from build123d import *

# Parameters (mm, degrees)
SKETCH_1_W          = 19
SKETCH_1_H          = 32
EXTRUDE_1_DEPTH     = 67
FILLET_1_R          = 1
SHELL_1_T           = 1.3
SKETCH_2_W          = 49
SKETCH_2_H          = 24
CUT_EXTRUDE_1_DEPTH = 74.32305231
CUT_EXTRUDE_2_REACH = 79.322
SKETCH_4_W          = 5.786103887
SKETCH_4_H          = 2
SKETCH_4_W_2        = 5.809063148
EXTRUDE_2_DEPTH     = 1.3


with BuildPart() as part:
    # 草图1 → 凸台-拉伸1 (new body)
    with BuildSketch(Plane(origin=(0, 0, 0), x_dir=(0, 0, -1), z_dir=(1, 0, 0))):
        Rectangle(SKETCH_1_W, SKETCH_1_H)
    extrude(amount=EXTRUDE_1_DEPTH)

    # 圆角1
    fillet_1_edges = [part.edges().sort_by_distance(p)[0] for p in [
        (67, -16, 0),
        (0, -16, 0),
        (0, 16, 0),
        (67, 16, 0),
    ]]
    fillet(fillet_1_edges, radius=FILLET_1_R)

    # 抽壳1
    shell_1_openings = [part.faces().sort_by_distance(p)[0] for p in [
        (33.5, 0, -9.5),
    ]]
    offset(amount=SHELL_1_T, openings=shell_1_openings, kind=Kind.INTERSECTION)

    # 草图2 → 切除-拉伸1 (cut, through all)
    with BuildSketch(Plane.XY.offset(10.8)):
        with Locations((32, 0)):
            Rectangle(SKETCH_2_W, SKETCH_2_H)
    extrude(amount=-CUT_EXTRUDE_1_DEPTH, mode=Mode.SUBTRACT)

    # 草图3 → 切除-拉伸2 (cut, up to next)
    with BuildSketch(Plane.XZ.offset(17.3), mode=Mode.PRIVATE) as cut_extrude_2_sk1:
        with BuildLine():
            Line((11.05, 2.9), (17.35, 2.9))
            ThreePointArc((17.35, 2.9), (19.1, 1.15), (17.35, -0.6))
            Line((17.35, -0.6), (11.05, -0.6))
            ThreePointArc((11.05, -0.6), (9.3, 1.15), (11.05, 2.9))
        make_face()
    cut_extrude_2_tool1 = extrude(cut_extrude_2_sk1.sketch, amount=-CUT_EXTRUDE_2_REACH, mode=Mode.PRIVATE) & part.part
    add(cut_extrude_2_tool1.solids().sort_by_distance((14.2, -17.3, 1.15))[0], mode=Mode.SUBTRACT)

    # 草图4 → 凸台-拉伸2 (add)
    with BuildSketch(Plane.XZ.offset(-16)):
        with Locations((10.323725872, 2)):
            Rectangle(SKETCH_4_W, SKETCH_4_H)
        with Locations((58.142746149, 2)):
            Rectangle(SKETCH_4_W_2, SKETCH_4_H)
    extrude(amount=EXTRUDE_2_DEPTH)


solid = part.part
Can you work these out from the model? Positions are in its coordinate system, mm. A direction names the side the tool comes from. Round coordinates to 2 decimals unless told otherwise and drop trailing zeros. Write each loop counter-clockwise with the first axis right and the second up, starting at its lowest first coordinate (ties: lowest second). Pieces come first, ordered by that corner, then holes. Notation, with made-up numbers: (69.5, 48) -> (110.5, 48) arc R17 ccw to (110.5, 53) -> close; hole circle Ø6 at (-9, 40.25). An arc over 180 degrees is marked (long way). Use one line per item in the form item = value. Start each with the question number.
Q1. Imagine slicing it at C-C (x = 62). Please give me the cut outline in (y, z), then the cut area to 3 significant figures.
Q2. We'd pull the mould along Y, two halves only. Please class faces 6 (the face through (10, 14.7, 2)), 7 (the face through (68.3, 0, 1)), 8 (the face through (33, -17.3, 1)): +Y half, -Y half, draft (parallel to the pull), parting line (faces both ways), or undercut.
Q3. Imagine slicing it at B-B (y = -9). Please give me the cut outline in (x, z).
Q4. If I drill on probe 1 along Y at (x, z) = (52, 10.25); probe 2 along Y at (x, z) = (14.5, -2.5); probe 3 along X at (y, z) = (7, -2.75), over which ranges is the centre line in solid material (lowest first)? Write a range as [from, to].
Q5. Imagine slicing it at D-D (z = 6.5). Please give me the cut outline in (x, y).
Q6. Imagine slicing it at A-A (x = 46). Please give me the cut outline in (y, z), then the cut area to 3 significant figures.
Q7. Which directions (+Z, -Z, +X, -X, +Y, -Y) give clear straight access to the entire face, cutting with the end or side of a thin tool? Please do faces 1 (the face through (32, -12, 10)), 2 (the face through (23, 17, -9.5)), 3 (the face through (33, 17.3, 1)), 4 (the face through (33, -16, 0)), 5 (the face through (14, -17, 2.9)).
Worked out:
q1.outline = (-17.3, -9.5) -> (-16, -9.5) -> (-16, 9.5) -> (16, 9.5) -> (16, -9.5) -> (17.3, -9.5) -> (17.3, 10.8) -> (-17.3, 10.8) -> close
q1.area = 94.4 mm^2
q2.face_6 = undercut
q2.face_7 = draft
q2.face_8 = -Y half
q3.outline = (-1.3, -9.5) -> (0, -9.5) -> (0, 9.5) -> (7.5, 9.5) -> (7.5, 10.8) -> (-1.3, 10.8) -> close; (56.5, 9.5) -> (67, 9.5) -> (67, -9.5) -> (68.3, -9.5) -> (68.3, 10.8) -> (56.5, 10.8) -> close
q4.probe_1 = [-17.3, -12], [12, 17.3]
q4.probe_2 = [-17.3, -16], [16, 17.3]
q4.probe_3 = [-1.3, 0], [67, 68.3]
q5.outline = (-1.3, -15) arc R2.3 ccw to (1, -17.3) -> (66, -17.3) arc R2.3 ccw to (68.3, -15) -> (68.3, 15) arc R2.3 ccw to (66, 17.3) -> (1, 17.3) arc R2.3 ccw to (-1.3, 15) -> close; hole (0, -15) arc R1 ccw to (1, -16) -> (66, -16) arc R1 ccw to (67, -15) -> (67, 15) arc R1 ccw to (66, 16) -> (1, 16) arc R1 ccw to (0, 15) -> close
q6.outline = (-17.3, -9.5) -> (-16, -9.5) -> (-16, 9.5) -> (-12, 9.5) -> (-12, 10.8) -> (-17.3, 10.8) -> close; (12, 9.5) -> (16, 9.5) -> (16, -9.5) -> (17.3, -9.5) -> (17.3, 10.8) -> (12, 10.8) -> close
q6.area = 63.2 mm^2
q7.face_1 = +Z, -Z
q7.face_2 = -Z, +X, -X, +Y, -Y
q7.face_3 = +Z, -Z, +X, -X, +Y
q7.face_4 = -Z
q7.face_5 = -Y
